Geometry check sheet. Reference: drawing and pictorial views, mm from the part's lowest x, y, z. Round coordinates to 2 decimals unless told otherwise and drop trailing zeros. Write each loop counter-clockwise with the first axis right and the second up, starting at its lowest first coordinate (ties: lowest second). Pieces come first, ordered by that corner, then holes. Notation, with made-up numbers: (21.5, 43) - (58.5, 43) arc R16 cw to (58.5, 62) - close; hole circle Ø2 at (-31.75, 88). An arc over 180 degrees is marked (long way). Return JSON: item names as keys, results as strings.
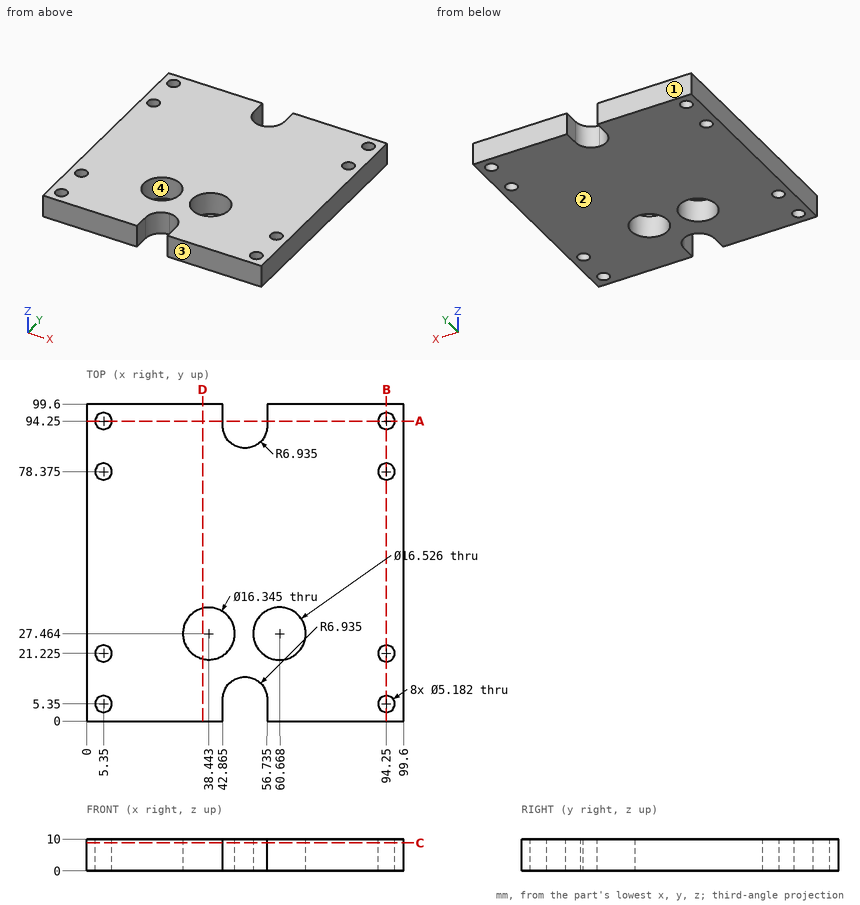
(1) Gauge pin test, flat end, axial feed: pin 1 (4.5 mm diameter, centred on x = 5.35, y = 5.35, fed in from -Z). Record the tip position at first contact, or that the pin passes through.
Response values:
{"pin 1": "passes through"}
(2) Section check D-D, the plane x = 36.5. Enter the section's corners in (y, z).
Response values:
{"outline": "(0, 0) - (19.53, 0) - (19.53, 10) - (0, 10) - close; (35.4, 0) - (99.6, 0) - (99.6, 10) - (35.4, 10) - close"}
(3) Material ranges on line 1 along Y through (x, z) = (94.25, 4) (1 decimal); line 2 along Y through (x, z) = (93, 2) (1 decimal); line 3 along X through (y, z) = (35, 4) (1 decimal), recorded low to high. Write a range as [from, to].
Response values:
{"line 1": "y = [0, 2.8], [7.9, 18.6], [23.8, 75.8], [81, 91.7], [96.8, 99.6]", "line 2": "y = [0, 3.1], [7.6, 19], [23.5, 76.1], [80.6, 92], [96.5, 99.6]", "line 3": "x = [0, 35.3], [41.6, 57.3], [64.1, 99.6]"}
(4) Section check B-B, the plane x = 94.25. Enter the section's corners in (y, z) (1 decimal).
Response values:
{"outline": "(0, 0) - (2.8, 0) - (2.8, 10) - (0, 10) - close; (7.9, 0) - (18.6, 0) - (18.6, 10) - (7.9, 10) - close; (23.8, 0) - (75.8, 0) - (75.8, 10) - (23.8, 10) - close; (81, 0) - (91.7, 0) - (91.7, 10) - (81, 10) - close; (96.8, 0) - (99.6, 0) - (99.6, 10) - (96.8, 10) - close"}
(5) Section check A-A, the plane y = 94.25. Enter the section's corners in (x, z) (1 decimal).
Response values:
{"outline": "(0, 0) - (2.8, 0) - (2.8, 10) - (0, 10) - close; (7.9, 0) - (42.9, 0) - (42.9, 10) - (7.9, 10) - close; (56.7, 0) - (91.7, 0) - (91.7, 10) - (56.7, 10) - close; (96.8, 0) - (99.6, 0) - (99.6, 10) - (96.8, 10) - close"}
(6) Section check C-C, the plane z = 8.75. Give the number of separate pieces and of enclosed holes in the cut face, plus the area to 3 significant figures.
Response values:
{"separate pieces": "1", "enclosed holes": "10", "area": "8,980 mm^2"}
(7) Release check for a two-part mould opening along Y. For the marked faces 1, 2, 3 and 4 record: pulls with the +Y half, pulls with the -Y half, needs draft (parallel to the pull), parting line crosses it, or undercut.
Response values:
{"face 1": "pulls with the +Y half", "face 2": "needs draft", "face 3": "pulls with the -Y half", "face 4": "undercut"}
